from build123d import *

# Parameters (mm, degrees)
SKETCH1_W           = 82.55
SKETCH1_H           = 65.0748
SKETCH1_W_2         = 69.85
SKETCH1_H_2         = 52.3748
BOSS_EXTRUDE1_DEPTH = 44.45
SKETCH2_W           = 184.15
SKETCH2_H           = 166.6748
BOSS_EXTRUDE4_DEPTH = 6.35
FILLET2_R           = 6.35
SKETCH3_R           = 3.175
CUT_EXTRUDE1_DEPTH  = 174.494911496
FILLET4_R           = 25.4
CUT_EXTRUDE2_DEPTH  = 174.494911496


with BuildPart() as part:
    # Sketch1 → Boss-Extrude1 (new body)
    with BuildSketch(Plane(origin=(0, 0, 0), x_dir=(1, 0, 0), z_dir=(0, 1, 0))):
        with Locations((34.925, 26.1874)):
            Rectangle(SKETCH1_W, SKETCH1_H)
        with Locations((34.925, 26.1874)):
            Rectangle(SKETCH1_W_2, SKETCH1_H_2, mode=Mode.SUBTRACT)
    extrude(amount=BOSS_EXTRUDE1_DEPTH)

    # Sketch2 → Boss-Extrude4 (add)
    with BuildSketch(Plane.XZ):
        with Locations((34.925, -26.1874)):
            Rectangle(SKETCH2_W, SKETCH2_H)
    extrude(amount=BOSS_EXTRUDE4_DEPTH)

    # Fillet2
    fillet2_edges = [part.edges().sort_by_distance(p)[0] for p in [
        (0, 22.225, -52.3748),
        (0, 22.225, 0),
        (69.85, 22.225, 0),
        (69.85, 22.225, -52.3748),
        (-57.15, -3.175, 57.15),
        (-57.15, -3.175, -109.5248),
        (127, -3.175, -109.5248),
        (127, -3.175, 57.15),
        (-6.35, 22.225, -58.7248),
        (76.2, 22.225, -58.7248),
        (76.2, 22.225, 6.35),
        (-6.35, 22.225, 6.35),
    ]]
    fillet(fillet2_edges, radius=FILLET2_R)

    # Sketch3 → Cut-Extrude1 (cut, through all)
    with BuildSketch(Plane(origin=(0, 0, 0), x_dir=(1, 0, 0), z_dir=(0, 1, 0))):
        with Locations(Location((104.670538096, 89.177877977, 0), (0, 0, 270))):
            Circle(SKETCH3_R)
        with Locations(Location((-34.820538096, -36.803077977, 0), (0, 0, 270))):
            Circle(SKETCH3_R)
        with Locations(Location((104.670538096, -36.803077977, 0), (0, 0, 270))):
            Circle(SKETCH3_R)
        with Locations(Location((-34.820538096, 89.177877977, 0), (0, 0, 270))):
            Circle(SKETCH3_R)
    extrude(amount=-CUT_EXTRUDE1_DEPTH, mode=Mode.SUBTRACT)

    # Fillet4
    fillet4_edges = [part.edges().sort_by_distance(p)[0] for p in [
        (-6.35, 0, -26.1874),
        (34.925, 0, -58.7248),
        (76.2, 0, -26.1874),
        (34.925, 0, 6.35),
        (-4.490128061, 0, -56.864928061),
        (-4.490128061, 0, 4.490128061),
        (74.340128061, 0, -56.864928061),
        (74.340128061, 0, 4.490128061),
    ]]
    fillet(fillet4_edges, radius=FILLET4_R)

    # Sketch4 → Cut-Extrude2 (cut, through all)
    with BuildSketch(Plane(origin=(0, 0, 0), x_dir=(1, 0, 0), z_dir=(0, 1, 0))):
        with BuildLine():
            Line((0, 46.0248), (0, 6.35))
            ThreePointArc((0, 6.35), (1.859871939, 1.859871939), (6.35, 0))
            Line((6.35, 0), (63.5, 0))
            ThreePointArc((63.5, 0), (67.990128061, 1.859871939), (69.85, 6.35))
            Line((69.85, 6.35), (69.85, 46.0248))
            ThreePointArc((69.85, 46.0248), (67.990128061, 50.514928061), (63.5, 52.3748))
            Line((63.5, 52.3748), (6.35, 52.3748))
            ThreePointArc((6.35, 52.3748), (1.859871939, 50.514928061), (0, 46.0248))
        make_face()
    extrude(amount=-CUT_EXTRUDE2_DEPTH, mode=Mode.SUBTRACT)


solid = part.part
Source: CAD feature listing. Evaluate the final solid. Frame: model axes, mm. A direction names the side the tool comes from. Give positions to 0.01 mm unless a question says otherwise; leave off trailing zeros. Write each loop counter-clockwise with the first axis right and the second up, starting at its lowest first coordinate (ties: lowest second). Pieces come first, ordered by that corner, then holes. Notation, with made-up numbers: (55, 76.5) -> (109, 76.5) arc R18 cw to (109, 103.5) -> close; hole circle Ø3 at (64.5, -17). An arc over 180 degrees is marked (long way). Return JSON: item names as keys, results as strings. Group by question number.
1. Section C-C, the plane x = 54. Output: boundary loops of the cut face in (y, z), then the cut area to 3 significant figures.
2. Access query for faces 4 (the face through (-4.54, 35.06, 4.44)), 5 (the face through (-4.539, 35.058, -56.815)), 6 (the face through (-6.35, 35, -26)). Directions: +Z, -Z, +X, -X, +Y, -Y. A direction counts if a zero-diameter tool reaches every point of the face in a straight line with its end or side. Return the directions, or none.
3. Section B-B, the plane z = -15. Output: boundary loops of the cut face in (x, y), then the cut area to 3 significant figures.
4. Section D-D, the plane y = 6.5. Output: boundary loops of the cut face in (x, z), then the cut area to 3 significant figures.
5. Section A-A, the plane y = 37.5. Output: boundary loops of the cut face in (x, z).
6. Pin query (flat end, axial travel): pin 1 Ø15 at (x, y) = (28, 36.5) entering from -Z; pin 2 Ø10 at (x, z) = (104.67, -89.18) entering from +Y; pin 3 Ø3 at (x, y) = (-4, 23.5) entering from +Z. Return the tip coordinate at first contact, or that it passes through.
7. Material intervals for line 1 (Z direction, x = 60, y = 35); line 2 (Y direction, x = -8, z = -87.5), sorted ascending. Write a range as from..to.
8. Mould query, pull axis X, two halves, no side actions, for faces 1 (the face through (74.29, 35.058, -56.914)), 2 (the face through (34.44, 7.24, 13.99)), 3 (the face through (35, 19, 0)). Classes: +X half, -X half, draft (parallel to the pull), parting line (faces both ways), or undercut.
Determined:
{
 "1": {"outline": "(-6.35, -109.52) -> (0, -109.52) -> (0, -84.12) arc R25.4 cw to (25.4, -58.72) -> (44.45, -58.72) -> (44.45, -52.37) -> (-6.35, -52.37) -> close; (-6.35, 0) -> (44.45, 0) -> (44.45, 6.35) -> (25.4, 6.35) arc R25.4 cw to (0, 31.75) -> (0, 57.15) -> (-6.35, 57.15) -> close", "area": "1,570 mm2"},
 "2": {"face 4": "+Z, -X, +Y", "face 5": "-Z, -X, +Y", "face 6": "+Z, -Z, -X, +Y"},
 "3": {"outline": "(-57.15, -6.35) -> (0, -6.35) -> (0, 44.45) -> (-6.35, 44.45) -> (-6.35, 25.4) arc R25.4 cw to (-31.75, 0) -> (-57.15, 0) -> close; (69.85, -6.35) -> (127, -6.35) -> (127, 0) -> (101.6, 0) arc R25.4 cw to (76.2, 25.4) -> (76.2, 44.45) -> (69.85, 44.45) -> close", "area": "1,570 mm2"},
 "4": {"outline": "(-14.78, -52.37) arc R14.78 ccw to (0, -67.16) -> (69.85, -67.16) arc R14.78 ccw to (84.63, -52.37) -> (84.63, 0) arc R14.78 ccw to (69.85, 14.78) -> (0, 14.78) arc R14.78 ccw to (-14.78, 0) -> close; hole (0, -46.02) arc R6.35 ccw to (6.35, -52.37) -> (63.5, -52.37) arc R6.35 ccw to (69.85, -46.02) -> (69.85, -6.35) arc R6.35 ccw to (63.5, 0) -> (6.35, 0) arc R6.35 ccw to (0, -6.35) -> close", "area": "4,330 mm2"},
 "5": {"outline": "(-6.35, -52.37) arc R6.35 ccw to (0, -58.72) -> (69.85, -58.72) arc R6.35 ccw to (76.2, -52.37) -> (76.2, 0) arc R6.35 ccw to (69.85, 6.35) -> (0, 6.35) arc R6.35 ccw to (-6.35, 0) -> close; hole (0, -46.02) arc R6.35 ccw to (6.35, -52.37) -> (63.5, -52.37) arc R6.35 ccw to (69.85, -46.02) -> (69.85, -6.35) arc R6.35 ccw to (63.5, 0) -> (6.35, 0) arc R6.35 ccw to (0, -6.35) -> close"},
 "6": {"pin 1": "stops at z = -58.72", "pin 2": "stops at y = 0", "pin 3": "stops at z = 5.93"},
 "7": {"line 1": "z = -58.72..-52.37, 0..6.35", "line 2": "y = -6.35..0"},
 "8": {"face 1": "+X half", "face 2": "draft", "face 3": "undercut"}
}
